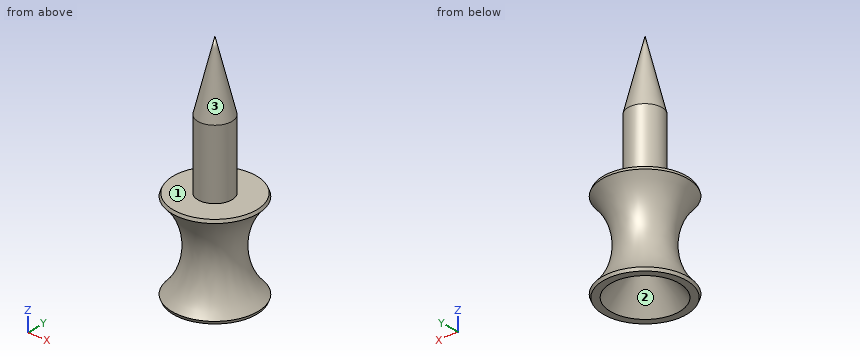
```python
from build123d import *


# Not quite as in the source:
# - a fillet or chamfer that OpenCascade refuses, or shapes differently, is made with other operations: its cross-section is extruded or revolved along the edge and cut away or added


with BuildPart() as f1:
    # F0 (on Front) → F1 (revolve)
    with BuildSketch(Plane.XZ):
        with BuildLine():
            Line((0, 31.75), (0, 6.35))
            Line((0, 6.35), (4.7625, 0))
            Line((4.7625, 0), (6.35, 0))
            ThreePointArc((6.35, 0), (3.4925, 6.35), (6.35, 12.7))
            Line((6.35, 12.7), (2.3495, 12.7))
            Line((2.3495, 12.7), (2.3495, 22.225))
            Line((2.3495, 22.225), (0, 31.75))
        make_face()
    revolve(axis=Axis((0, 0, 19.05), (0, 0, -1)))

    # F2: chamfer of 0.635 on 2 edges, made by hand

    # F2_s1 → F2_t2 (revolve, cut)
    with BuildSketch(Plane.XZ):
        with BuildLine():
            Line((5.929083675, 12.2670736629), (5.7374458679, 12.7234188432))
            Line((5.7374458679, 12.7234188432), (5.7374458679, 12.7361188432))
            ThreePointArc((5.7374458679, 12.7361188432), (6.043722934, 12.7127), (6.35, 12.7127))
            Line((6.35, 12.7127), (6.3584226611, 12.6904948025))
            ThreePointArc((6.3584226611, 12.6904948025), (6.1365228233, 12.4867090771), (5.9381511191, 12.2581814496))
            Line((5.9381511191, 12.2581814496), (5.929083675, 12.2670736629))
        make_face()
    revolve(axis=Axis((0, 0, 12.7), (0, 0, -1)), mode=Mode.SUBTRACT)

    # F2_s3 → F2_t4 (revolve, cut)
    with BuildSketch(Plane.XZ):
        with BuildLine():
            Line((5.7374458679, -0.0234188432), (5.929083675, 0.4329263371))
            Line((5.929083675, 0.4329263371), (5.9381511191, 0.4418185504))
            ThreePointArc((5.9381511191, 0.4418185504), (6.1365228233, 0.2132909229), (6.3584226611, 0.0095051975))
            Line((6.3584226611, 0.0095051975), (6.35, -0.0127))
            ThreePointArc((6.35, -0.0127), (6.043722934, -0.0127), (5.7374458679, -0.0361188432))
            Line((5.7374458679, -0.0361188432), (5.7374458679, -0.0234188432))
        make_face()
    revolve(axis=Axis((0, 0, 0), (0, 0, -1)), mode=Mode.SUBTRACT)


solid = f1.part
```
Part model, mm, in its own coordinate system. Face numbers are marked on the shaded views. Coordinates: 2 decimals unless noted, no trailing zeros. Order: outer loops, then holes, each group sorted by start corner. A loop starts at its lowest first (then second) coordinate and runs counter-clockwise, first axis right, second up. Notation, with made-up numbers: (-36.75, -16) -> (14.25, -16) arc R26 cw to (14.25, 6) -> close; hole circle Ø6 at (-24, 34). An arc over 180 degrees is marked (long way). Put each result on its own line as item: value. Start each with the question number.
(1) Pin check, flat tips, straight feed: pin 1 Ø1.5 at (x, z) = (1.5, 19.5) entering from -Y; pin 2 Ø2 at (x, y) = (2.5, -4) entering from +Z; pin 3 Ø5 at (y, z) = (-0.5, 27) entering from -X. Stop position of each tip, or through.
(2) Probe line 1 along Z through (x, y) = (-4.25, 1); line 2 along Z through (x, y) = (-2.75, 4.75); line 3 along X through (y, z) = (-0.5, 14.5). List the from-to ranges inside material, lowest first. Write a range as [from, to].
(3) Band-saw the part on B-B (z = 4). Give the cut face in (x, y) (1 decimal), then the cut area to 3 significant figures.
(4) Band-saw the part on A-A (z = 11). Give the cut face in (x, y).
(5) Band-saw the part on C-C (z = 27). Give the cut face in (x, y).
(6) Mould opens along X. For the marked faces 1, 2 and 3 say: pulls with the +X half, pulls with the -X half, needs draft (parallel to the pull), parting line crosses it, or undercut.
Determined:
1. pin 1: stops at y = -2.23
1. pin 2: stops at z = 12.7
1. pin 3: stops at x = -1.78
2. line 1: z = [0.53, 2.6], [10.1, 12.7]
2. line 2: z = [0, 0.88], [11.82, 12.7]
2. line 3: x = [-2.3, 2.3]
3. outline: circle Ø7.6 at (0, 0); hole circle Ø3.5 at (0, 0)
3. area: 36.2 mm²
4. outline: circle Ø9.76 at (0, 0)
5. outline: circle Ø2.34 at (0, 0)
6. face 1: needs draft
6. face 2: undercut
6. face 3: parting line crosses it
